```python
from build123d import *

# Parameters (mm, degrees)
SKETCH1_W     = 240
SKETCH1_H     = 7.5
CHAMFER1_SIZE = 0.5


with BuildPart() as part:
    # Sketch1 → Revolve1 (revolve)
    with BuildSketch(Plane.XY, mode=Mode.PRIVATE) as revolve1_sk:
        with Locations((120, 3.75)):
            Rectangle(SKETCH1_W, SKETCH1_H)
    revolve(revolve1_sk.sketch.rotate(Axis((0, 0, 0), (1, 0, 0)), 180), axis=Axis((0, 0, 0), (1, 0, 0)))

    # Sketch2 → Cut-Revolve1 (revolve, cut)
    with BuildSketch(Plane.XY, mode=Mode.PRIVATE) as cut_revolve1_sk:
        Polygon((0, 0.5), (0, 0), (0.5, 0), align=None)
        Polygon((239.5, 0), (240, 0.5), (240, 0), align=None)
    revolve(cut_revolve1_sk.sketch.rotate(Axis((0, 0, 0), (1, 0, 0)), 90), axis=Axis((0, 0, 0), (1, 0, 0)), mode=Mode.SUBTRACT)

    # Chamfer1
    chamfer1_edges = [part.edges().sort_by_distance(p)[0] for p in [
        (0, 7.5, 0),
        (240, 7.5, 0),
    ]]
    chamfer(chamfer1_edges, length=CHAMFER1_SIZE)


solid = part.part
```
Read the model definition and answer for the solid it produces. Units are mm, in the model's axes. Give positions to 0.01 mm unless a question says otherwise; leave off trailing zeros. Loops run counter-clockwise (first coordinate to the right, second up) from the corner with the lowest first, then second, coordinate; pieces in that order, holes last.
Item 1: Find the intervals of material crossed by line 1 along Y through (x, z) = (124, -2.75); line 2 along Y through (x, z) = (75.5, -0.5); line 3 along Z through (x, y) = (173, -0.75), in increasing order.
Item 2: The part is cut by section A-A (x = 93). Write down the section's boundary in (y, z), and give its area (3 significant figures).
Item 3: Each of these flat-tipped pins is pushed along its axis until it touches: pin 1 Ø1 at (x, y) = (76, 5) entering from -Z; pin 2 Ø2 at (x, y) = (156, -3) entering from +Z; pin 3 Ø3 at (x, z) = (141.5, 3.5) entering from -Y. Where does it stop, or does it pass through?
Taken from the geometry:
1. line 1: y = -6.98 to 6.98
1. line 2: y = -7.48 to 7.48
1. line 3: z = -7.46 to 7.46
2. outline: circle Ø15 at (0, 0)
2. area: 177 mm2
3. pin 1: stops at z = -6
3. pin 2: stops at z = 7.23
3. pin 3: stops at y = -7.23
